Could you check a few things on this model? Use its own coordinates, in mm. A direction names the side the tool comes from. Coordinates: 2 decimals unless noted, no trailing zeros. Order: outer loops, then holes, each group sorted by start corner. A loop starts at its lowest first (then second) coordinate and runs counter-clockwise, first axis right, second up. Notation, with made-up numbers: (30.25, -15.5) - (61.25, -15.5) arc R11 ccw to (61.25, 3.5) - close; hole circle Ø11 at (80, 0). An arc over 180 degrees is marked (long way). Answer as a JSON object with one key per item and string values. Group by question number.
(1) Imagine slicing it at D-D, the plane y = 35.75. Give the number of separate pieces and of enclosed holes in the cut face, and give its area (3 significant figures).
(2) Imagine slicing it at C-C, the plane x = 0. Write out the boundary of the cut face in (y, z).
(3) Imagine slicing it at B-B, the plane y = 19. Write out the boundary of the cut face in (x, z), and give its area (3 significant figures).
(4) Please list where these lines run through material, in increasing order: probe 1 along X at (y, z) = (37.5, 9.5); probe 2 along Y at (x, z) = (35.75, 3.85); probe 3 along Y at (x, z) = (35.75, 2.15).
(5) Imagine slicing it at A-A, the plane z = 1.75. Write out the boundary of the cut face in (x, y).
(6) Which directions (+Z, -Z, +X, -X, +Y, -Y) give clear straight access to the entire face, cutting with the end or side of a thin tool? Please do faces 3 (the flat face through (38, 36, 5)), 4 (the flat face through (-9, -39, 8)), 5 (the flat face through (-1, 41.75, 6)), 6 (the cylindrical face through (-37.2, -36.9, 6.5)).
(7) We'd pull the mould along X, two halves only. Please class faces 1 (the cylindrical face through (-37.2, 34.6, 6.5)), 2 (the flat face through (-1, 49, 1)): pulls with the +X half, pulls with the -X half, needs draft (parallel to the pull), parting line crosses it, or undercut.
(8) Will these pins go through, and if not, where does the flat tip stop? P1, Ø3, axis at x = 35.75, y = -35.75, coming from the -Z side; P2, Ø2, axis at y = -1.5, z = 6.5, coming from the -X side; P3, Ø0.6, axis at x = 0.5, z = 8.5, coming from the +Y side; P4, Ø5, axis at x = 35.75, y = -35.75, coming from the -Z side.
from build123d import *

# Parameters (mm, degrees)
SKETCH_W        = 98
SKETCH_H        = 98
PAD_DEPTH       = 3
SKETCH001_W     = 83.5
SKETCH001_H     = 83.5
PAD001_DEPTH    = 7
SKETCH002_R     = 39.5
POCKET_DEPTH    = 10
SKETCH003_W     = 80.5
SKETCH003_H     = 80.5
POCKET001_DEPTH = 2
SKETCH004_R     = 1.85
POCKET002_DEPTH = 8
SKETCH005_R     = 2.75
POCKET003_DEPTH = 5
CHAMFER_SIZE    = 0.5


with BuildPart() as part:
    # Sketch → Pad (new body)
    with BuildSketch(Plane.XY):
        Rectangle(SKETCH_W, SKETCH_H)
    extrude(amount=PAD_DEPTH)

    # Sketch001 (on Face6 of Pad) → Pad001 (join)
    with BuildSketch(Plane.XY.offset(3)):
        Rectangle(SKETCH001_W, SKETCH001_H)
    extrude(amount=PAD001_DEPTH)

    # Sketch002 (on Face11 of Pad001) → Pocket (cut)
    with BuildSketch(Plane.XY.offset(10)):
        Circle(SKETCH002_R)
    extrude(amount=-POCKET_DEPTH, mode=Mode.SUBTRACT)

    # Sketch003 (on Face12 of Pocket) → Pocket001 (cut)
    with BuildSketch(Plane.XY.offset(10)):
        Rectangle(SKETCH003_W, SKETCH003_H)
    extrude(amount=-POCKET001_DEPTH, mode=Mode.SUBTRACT)

    # Sketch004 (on Face12 of Pocket001) → Pocket002 (cut)
    with BuildSketch(Plane.XY.offset(8)):
        with Locations((-35.75, 35.75)):
            Circle(SKETCH004_R)
        with Locations((35.75, 35.75)):
            Circle(SKETCH004_R)
        with Locations((35.75, -35.75)):
            Circle(SKETCH004_R)
        with Locations((-35.75, -35.75)):
            Circle(SKETCH004_R)
    extrude(amount=-POCKET002_DEPTH, mode=Mode.SUBTRACT)

    # Sketch005 (on Face4 of Pocket002) → Pocket003 (cut)
    with BuildSketch(Plane(origin=(0, 0, 0), x_dir=(1, 0, 0), z_dir=(0, 0, -1))):
        with Locations((-35.75, 35.75)):
            Circle(SKETCH005_R)
        with Locations((35.75, 35.75)):
            Circle(SKETCH005_R)
        with Locations((35.75, -35.75)):
            Circle(SKETCH005_R)
        with Locations((-35.75, -35.75)):
            Circle(SKETCH005_R)
    extrude(amount=-POCKET003_DEPTH, mode=Mode.SUBTRACT)

    # Chamfer
    chamfer_edges = [part.edges().sort_by_distance(p)[0] for p in [
        (33, 35.75, 0),
        (33, -35.75, 0),
        (-38.5, -35.75, 0),
        (-38.5, 35.75, 0),
    ]]
    chamfer(chamfer_edges, length=CHAMFER_SIZE)


solid = part.part
Result set:
{
 "1": {"separate pieces": "4", "enclosed holes": "0", "area": "371 mm^2"},
 "2": {"outline": "(-49, 0) - (-39.5, 0) - (-39.5, 8) - (-40.25, 8) - (-40.25, 10) - (-41.75, 10) - (-41.75, 3) - (-49, 3) - close; (39.5, 0) - (49, 0) - (49, 3) - (41.75, 3) - (41.75, 10) - (40.25, 10) - (40.25, 8) - (39.5, 8) - close"},
 "3": {"outline": "(-49, 0) - (-34.63, 0) - (-34.63, 8) - (-40.25, 8) - (-40.25, 10) - (-41.75, 10) - (-41.75, 3) - (-49, 3) - close; (34.63, 0) - (49, 0) - (49, 3) - (41.75, 3) - (41.75, 10) - (40.25, 10) - (40.25, 8) - (34.63, 8) - close", "area": "163 mm^2"},
 "4": {"probe 1": "x = -41.75 to -40.25, 40.25 to 41.75", "probe 2": "y = -41.75 to -38.5, -33 to -16.8, 16.8 to 33, 38.5 to 41.75", "probe 3": "y = -49 to -38.5, -33 to -16.8, 16.8 to 33, 38.5 to 49"},
 "5": {"outline": "(-49, -49) - (49, -49) - (49, 49) - (-49, 49) - close; hole circle Ø79 at (0, 0); hole circle Ø5.5 at (-35.75, -35.75); hole circle Ø5.5 at (-35.75, 35.75); hole circle Ø5.5 at (35.75, -35.75); hole circle Ø5.5 at (35.75, 35.75)"},
 "6": {"face 3": "-Z", "face 4": "+Z", "face 5": "+Z, +X, -X, +Y", "face 6": "+Z, -Z"},
 "7": {"face 1": "undercut", "face 2": "needs draft"},
 "8": {"P1": "passes through", "P2": "stops at x = -41.75", "P3": "stops at y = 41.75", "P4": "stops at z = 5"}
}
